Part model, mm, in its own coordinate system. Face numbers are marked on the shaded views. A direction names the side the tool comes from. Coordinates: 2 decimals unless noted, no trailing zeros. Write each loop counter-clockwise with the first axis right and the second up, starting at its lowest first coordinate (ties: lowest second). Pieces come first, ordered by that corner, then holes. Notation, with made-up numbers: M 63,56 L 70,56 A11 ccw 70,77 Z; hole C 28,45 d5. An arc over 180 degrees is marked long. Use a Markdown table: item, result. Add a question column.
Q1. Pin check, flat tips, straight feed: pin 1 Ø5 at (x, z) = (10, 4.5) entering from +Y; pin 2 Ø5 at (y, z) = (4.5, 4) entering from +X; pin 3 Ø8.5 at (x, z) = (9, 6.5) entering from +Y. Stop position of each tip, or through.
Q2. Wall check: L1, parallel to X at y = 0, z = 14.75; L2, parallel to X at y = -0.9, z = 4.5; L3, parallel to Z at x = 0, y = 3.6. Give the ranges that are in metal, low to high. Write a range as from..to.
Q3. Slice it at B-B on y = -1.5. Write the cut outline in (x, z), then the cut area to 3 significant figures.
Q4. Slice it at C-C on x = 0. Write the cut outline in (y, z).
Q5. Mould opens along Z. For the marked faces 1, 2 and 3 say: released by +Z, released by -Z, zero draft, split by the parting line, or undercut.
Q6. Slice it at A-A on x = -10. Write the cut outline in (y, z).
Q7. Tool access for the marked faces 4, 5, 6 and 7: list every direction of +Z, -Z, +X, -X, +Y, -Y with a clear straight run to the whole face (end or side of a thin tool).
Q8. Slice it at D-D on z = 14. Write the cut outline in (x, y), then the cut area to 3 significant figures.
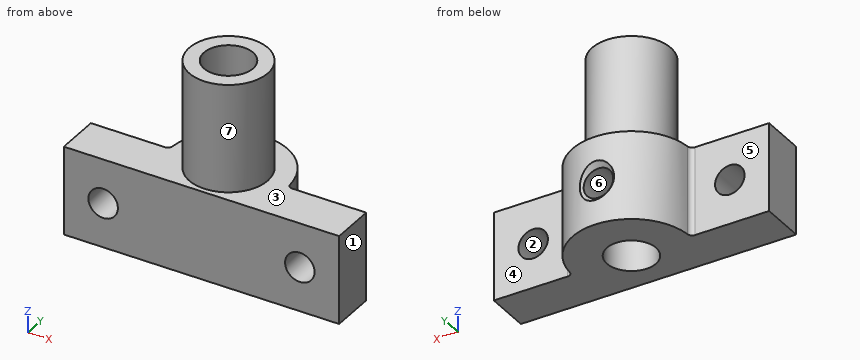
Autodesk Inventor part; units mm, degrees
ref_plane "YZ Plane" through (0, 0, 0) normal (1, 0, 0) x (0, 1, 0)
ref_plane "XZ Plane" through (0, 0, 0) normal (0, 1, 0) x (-1, 0, 0)
ref_plane "XY Plane" through (0, 0, 0) normal (0, 0, 1) x (1, 0, 0)
sketch "Sketch1" plane through (0, 0, 0) normal (0, 0, 1) x (1, 0, 0)
  line L0 (14, 0) -> (-14, 0)
  line L1 (-14, 0) -> (-14, -4.5)
  line L2 (-14, -4.5) -> (14, -4.5)
  line L3 (14, -4.5) -> (14, 0)
  line L4 (0, 29.3592) -> (0, -29.3592) construction
  arc A0 (5.9822, 0.4615) -> (-5.9822, 0.4615) centre (0, 0) ccw
  circle A1 centre (0, 0) radius 2.5
  circle A2 centre (0, 0) radius 4
  arc A3 (5.9822, 0.4615) -> (6.4807, 0) centre (6.4807, 0.5) ccw
  arc A4 (-6.4807, 0) -> (-5.9822, 0.4615) centre (-6.4807, 0.5) ccw
  dimension "d0" = 14
  dimension "d1" = 4.5
  dimension "d2" = 12
  dimension "d3" = 8
  dimension "d4" = 5
  dimension "d5" = 1
  dimension "d6" = 1
extrude "Extrusion1" add sketch "Sketch1" along normal blind 9 contours L3 L2 L1 L0 A2 | L0 A2 A4 A0 A3
extrude "Extrusion2" add sketch "Sketch1" along normal blind 20 contours A2 L0 A1 | L0 A1 A2
ref_plane "Plano de trabajo2" through (-14, 6, 0) normal (0, 1, 0) x (1, 0, 0)
sketch "Boceto3" plane through (-14, 6, 0) normal (0, 1, 0) x (1, 0, 0)
  line L0 (14, 0) -> (14, -9) construction
  line L1 (8.0178, -9) -> (19.9822, -9)
  line L2 (0, 0) -> (0, -9)
  line L3 (0, -4.5) -> (28, -4.5) construction
  line L4 (28, 0) -> (28, -9)
  circle A0 centre (4, -4.5) radius 1.5
  circle A1 centre (14, -4.5) radius 1.5
  circle A2 centre (24, -4.5) radius 1.5
  line L5 (7.5193, 0) -> (0, 0)
  line L6 (0, 0) -> (0, -9)
  line L7 (7.5193, -9) -> (0, -9)
  line L8 (7.5193, 0) -> (7.5193, -9)
  line L9 (19.9822, 0) -> (8.0178, 0)
  line L10 (8.0178, 0) -> (8.0178, -9)
  line L11 (19.9822, -9) -> (8.0178, -9)
  line L12 (19.9822, 0) -> (19.9822, -9)
  line L13 (28, 0) -> (20.4807, 0)
  line L14 (20.4807, 0) -> (20.4807, -9)
  line L15 (28, -9) -> (20.4807, -9)
  line L16 (28, 0) -> (28, -9)
  dimension "d25" = 3
  dimension "d26" = 3
  dimension "d27" = 3
  dimension "d28" = 10
  dimension "d29" = 10
hole "Agujero2" at (0, 6, 4.5) direction (0, -1, 0) diameter 3 depth 5 countersink diameter 4 countersink angle 90
hole "Agujero3" at (-10, 6, 4.5) at (10, 6, 4.5) direction (0, -1, 0) diameter 3 end through all
properties part number "Hudson 1-71"
Recorded:
| question | item | result |
|---|---|---|
| 1 | pin 1 | y = 0 |
| 1 | pin 2 | x = 5.66 |
| 1 | pin 3 | y = 3.67 |
| 2 | L1 | -4..-2.5, 2.5..4 |
| 2 | L2 | -14..-11.5, -8.5..-2.33, 2.33..8.5, 11.5..14 |
| 2 | L3 | 0..3, 6..20 |
| 3 | outline | M -14,0 L -2,0 L -2,20 L -3.71,20 L -3.71,9 L -14,9 Z; M 2,0 L 14,0 L 14,9 L 3.71,9 L 3.71,20 L 2,20 Z; hole C -10,4.5 d3; hole C 10,4.5 d3 |
| 3 | area | 239 mm² |
| 4 | outline | M -4.5,0 L -2.5,0 L -2.5,20 L -4,20 L -4,9 L -4.5,9 Z; M 2.5,0 L 6,0 L 6,2.5 L 5.5,3 L 2.5,3 Z; M 2.5,6 L 5.5,6 L 6,6.5 L 6,9 L 4,9 L 4,20 L 2.5,20 Z |
| 5 | face 1 | zero draft |
| 5 | face 2 | undercut |
| 5 | face 3 | released by +Z |
| 6 | outline | M -4.5,0 L 0,0 L 0,3 L -4.5,3 Z; M -4.5,6 L 0,6 L 0,9 L -4.5,9 Z |
| 7 | face 4 | +Z, -Z, +X, +Y |
| 7 | face 5 | +Z, -Z, -X, +Y |
| 7 | face 6 | +Y |
| 7 | face 7 | +Z |
| 8 | outline | C 0,0 d8; hole C 0,0 d5 |
| 8 | area | 30.6 mm² |
